Part model, mm, in its own coordinate system. A direction names the side the tool comes from. Round coordinates to 2 decimals unless told otherwise and drop trailing zeros. Write each loop counter-clockwise with the first axis right and the second up, starting at its lowest first coordinate (ties: lowest second). Pieces come first, ordered by that corner, then holes. Notation, with made-up numbers: (-21, 68) -> (-9, 68) arc R10 ccw to (-9, 83) -> close; hole circle Ø1 at (73, -17.5). An arc over 180 degrees is marked (long way). Return JSON: item names as keys, results as strings. Group by question number.
(1) Tool access for faces 1 (the flat face through (-14.3, -0.1, 1.6)), 2 (the flat face through (-15, 2, 15)), 3 (the flat face through (0, 13, 13)), 4 (the flat face through (-14, 3.5, 15)), 5 (the conical face through (13.103, -2.91, 6.628)): list every direction of +Z, -Z, +X, -X, +Y, -Y with a clear straight run to the whole face (end or side of a thin tool).
(2) Mould opens along Y. For faces 6 (the flat face through (15, 2, 15)), 7 (the cylindrical face through (9.139, -14.334, 0.818)), 8 (the cylindrical face through (-9.766, -12.737, 0.789)), 9 (the flat face through (14, 5, 12)) say: +Y half, -Y half, draft (parallel to the pull), parting line (faces both ways), or undercut.
(3) Saw through at A-A (z = 14). List the corners of the cut face in (x, y).
(4) Drop flat-ended pins along their axis: pin 1 Ø1.4 at (x, z) = (-13, 13.5) entering from +Y; pin 2 Ø0.8 at (x, z) = (-14.5, 12.5) entering from -Y; pin 3 Ø4 at (x, y) = (4.5, 8.5) entering from +Z; pin 4 Ø1.5 at (x, y) = (12.5, 5) entering from +Z. Give the stop position or say it passes through.
(5) Drill centre lines: L1, parallel to Y at x = 0, z = 0.85; L2, parallel to Y at x = -2, z = 1.75. Where is each one in solid material? Low to high. Write a range as from..to.
Autodesk Inventor part; units mm, degrees
ref_plane "YZ Plane" through (0, 0, 0) normal (1, 0, 0) x (0, 1, 0)
ref_plane "XZ Plane" through (0, 0, 0) normal (0, 1, 0) x (-1, 0, 0)
ref_plane "XY Plane" through (0, 0, 0) normal (0, 0, 1) x (1, 0, 0)
sketch "Náčrt1" plane through (0, 0, 0) normal (0, 0, 1) x (1, 0, 0)
  circle A0 centre (0, 0) radius 17
  circle A1 centre (0, 0) radius 12.5
  line L0 (-2.5, -12.5) -> (2.5, -12.5)
  line L1 (2.5, -12.5) -> (2.5, 12.5)
  line L2 (2.5, 12.5) -> (-2.5, 12.5)
  line L3 (-2.5, 12.5) -> (-2.5, -12.5)
  line L4 (-2.5, -12.5) -> (2.5, 12.5) construction
  line L5 (2.5, -12.5) -> (-2.5, 12.5) construction
  line L6 (-12.5, -2.5) -> (12.5, -2.5)
  line L7 (12.5, -2.5) -> (12.5, 2.5)
  line L8 (12.5, 2.5) -> (-12.5, 2.5)
  line L9 (-12.5, 2.5) -> (-12.5, -2.5)
  line L10 (-12.5, -2.5) -> (12.5, 2.5) construction
  line L11 (12.5, -2.5) -> (-12.5, 2.5) construction
  dimension "d0" = 34
  dimension "d3" = 25
  dimension "d29" = 5
  dimension "d30" = 25
  dimension "d31" = 25
  dimension "d32" = 5
extrude "Vysunutí1" add sketch "Náčrt1" along normal blind 13 contours A0 | L7 L6 A1 | A1 L8 L7 | A1 L2 L1 | L1 L0 A1 | A1 L3 L2 | L0 L3 A1 | A1 L9 L8 | L6 L9 A1
sketch "Náčrt2" plane through (0, 0, 0) normal (1, 0, 0) x (0, 1, 0)
  line L0 (17, 0) -> (-17, 0)
  line L1 (17, 13) -> (-17, 13)
  line L2 (17, 0) -> (-17, 0)
  line L3 (-12.5, 13) -> (12.5, 13)
  line L4 (-12.5, 0) -> (12.5, 0)
  line L5 (17, 0) -> (17, 13)
  line L6 (12.5, 13) -> (12.5, 0)
  line L7 (0, -4.52) -> (0, 15.92)
  line L8 (16.05, -1.6) -> (13.95, -1.6)
  line L9 (13.95, -1.6) -> (13.95, 1.6)
  line L10 (13.95, 1.6) -> (16.05, 1.6)
  line L11 (16.05, 1.6) -> (16.05, -1.6)
  line L12 (16.05, -1.6) -> (13.95, 1.6) construction
  line L13 (13.95, -1.6) -> (16.05, 1.6) construction
  point P0 (0, 0)
  point P1 (15, 0)
  point P2 (13.95, 0)
  point P3 (16.05, 0)
  dimension "d36" = 2.1
  dimension "d37" = 1.6
  dimension "d38" = 2
  dimension "d39" = 2.5
revolve "Rotace1" cut sketch "Náčrt2" angle 360 about axis through (0, 0, -10) along (0, 0, 1) contours L0 L9 L10 L11
sketch "Náčrt4" plane through (0, 0, 13) normal (0, 0, 1) x (1, 0, 0)
  line L0 (-17, 6.5) -> (17, 6.5)
  line L1 (17, 6.5) -> (17, 3.5)
  line L2 (17, 3.5) -> (-17, 3.5)
  line L3 (-17, 3.5) -> (-17, 6.5)
  line L4 (-17, 6.5) -> (17, 3.5) construction
  line L5 (17, 6.5) -> (-17, 3.5) construction
  point P0 (0, 0)
  point P1 (0, 5)
  dimension "d9" = 3
  dimension "d10" = 34
  dimension "d11" = 5
extrude "Vysunutí2" cut sketch "Náčrt4" against normal blind 1
sketch "Náčrt5" plane through (0, 0, 0) normal (1, 0, 0) x (0, 1, 0)
  line L0 (17, 0) -> (17, 13)
  line L1 (17, 2) -> (13.2, 3.5)
  line L2 (17, 2) -> (21.0853, 2) construction
  line L3 (17, 0) -> (-17, 0)
  line L4 (13.2, 3.5) -> (13.2, 6.5)
  line L5 (17, 2) -> (17, 8.6939)
  line L6 (17, 8.6939) -> (13.2, 6.5)
  line L7 (0, -2.6) -> (0, 15.6)
  point P0 (0, 0)
  point P1 (0, 0)
  dimension "d15" = 2
  dimension "d16" = 13.2
  dimension "d17" = 60
  dimension "d20" = 3.5
  dimension "d21" = 68.459
  dimension "d22" = 3
revolve "Rotace2" cut sketch "Náčrt5" angle 360 about axis through (0, 0, -10) along (0, 0, 1)
fillet "Zaoblení1" radius 0.5 4 edges at (12.0208, 12.0208, 8.6939) (-12.0208, -12.0208, 8.6939) (-12.0208, -12.0208, 2) (12.0208, 12.0208, 2)
sketch "Náčrt6" plane through (0, 0, 13) normal (0, 0, 1) x (1, 0, 0)
  circle A0 centre (0, 0) radius 17
  circle A1 centre (0, 0) radius 12.5
  line L0 (17.5, -2) -> (-17.5, -2)
  line L1 (-17.5, -2) -> (-17.5, 2)
  line L2 (-17.5, 2) -> (17.5, 2)
  line L3 (17.5, 2) -> (17.5, -2)
  line L4 (17.5, -2) -> (-17.5, 2) construction
  line L5 (-17.5, -2) -> (17.5, 2) construction
  line L6 (17.5, -3.5) -> (-17.5, -3.5)
  line L7 (-17.5, -3.5) -> (-17.5, 3.5)
  line L8 (-17.5, 3.5) -> (17.5, 3.5)
  line L9 (17.5, 3.5) -> (17.5, -3.5)
  line L10 (17.5, -3.5) -> (-17.5, 3.5) construction
  line L11 (-17.5, -3.5) -> (17.5, 3.5) construction
  point P0 (12, 3.5)
  point P1 (16.6358, 3.5)
  point P2 (16.8819, 2)
  point P3 (12.339, 2)
  point P4 (-16.6358, 3.5)
  point P5 (-12, 3.5)
  point P6 (-12.339, 2)
  point P7 (-16.8819, 2)
  point P8 (-16.6358, 3.5)
  dimension "d23" = 35
  dimension "d25" = 35
  dimension "d26" = 4
  dimension "d33" = 7
extrude "Vysunutí4" add sketch "Náčrt6" along normal blind 4 contours L2 A1 L8 A0 | L8 A1 L2 A0
properties part number "sonar_3D tisk"
Computed values:
{
 "1": {"face 1": "-Z", "face 2": "+Z, +X, -X, -Y", "face 3": "+Z, +X, -X, +Y", "face 4": "+Z, +X, -X", "face 5": "none"},
 "2": {"face 6": "-Y half", "face 7": "parting line", "face 8": "undercut", "face 9": "undercut"},
 "3": {"outline": "(-16.88, 2) -> (-12.34, 2) arc R12.5 cw to (-12, 3.5) -> (-16.64, 3.5) arc R17 ccw to start; (12, 3.5) arc R12.5 cw to (12.34, 2) -> (16.88, 2) arc R17 ccw to (16.64, 3.5) -> close"},
 "4": {"pin 1": "y = 11.51", "pin 2": "y = -9.5", "pin 3": "through", "pin 4": "z = 12"},
 "5": {"L1": "-17..-16.05, -13.95..-12.5, 12.5..13.95, 16.05..17", "L2": "-16.87..-12.34, 12.34..16.87"}
}
